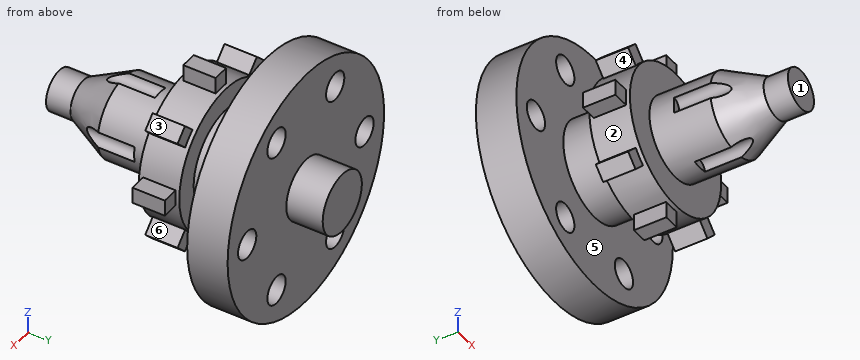
from build123d import *

# Parameters (mm, degrees)
HOLE2_START        = 255
HOLE2_OUTLINE_R    = 17.5
HOLE2_DEPTH        = 50
CIRPATTERN1_COUNT  = 6
RIB2_START         = -20
RIB2_DEPTH         = 40
CIRPATTERN2_COUNT  = 8
SKETCH13_R         = 10
CUT_EXTRUDE1_DEPTH = 125
CIRPATTERN3_COUNT  = 4


# Read off the part's stored shape, not the designer's step: Hole2, Rib2
with BuildPart() as part:
    # Sketch1 → Revolve1 (revolve)
    with BuildSketch(Plane.XY):
        Polygon((0, 0), (0, 350), (37.5, 350), (37.5, 305), (150, 305), (150, 255), (60, 255), (60, 205), (87.5, 205), (87.5, 155), (50, 155), (50, 80), (25, 30), (25, 0), align=None)
    revolve(axis=Axis((0, 0, 0), (0, 1, 0)))

    # Hole2 outline → Hole2 (cut)
    with BuildSketch(Plane(origin=(0, 0, 0), x_dir=(1, 0, 0), z_dir=(0, 1, 0)).offset(HOLE2_START)):
        with Locations((112.5, 0)):
            Circle(HOLE2_OUTLINE_R)
    hole2 = extrude(amount=HOLE2_DEPTH, mode=Mode.SUBTRACT)

    # CirPattern1: Hole2 ×6 about axis
    cirpattern1_axis = Axis((0, 0, 0), (0, 1, 0))
    for i in range(1, CIRPATTERN1_COUNT):
        add(hole2.rotate(cirpattern1_axis, i * 360 / CIRPATTERN1_COUNT), mode=Mode.SUBTRACT)

    # Rib2 outline → Rib2 (add)
    with BuildSketch(Plane(origin=(0, 180, 0), x_dir=(-1, 0, 0), z_dir=(0, -1, 0)).offset(RIB2_START)):
        with BuildLine():
            ThreePointArc((-10, 86.926693254), (0, 87.5), (10, 86.926693254))
            Line((10, 86.926693254), (10, 107.5))
            Line((10, 107.5), (-10, 107.5))
            Line((-10, 107.5), (-10, 86.926693254))
        make_face()
    rib2 = extrude(amount=RIB2_DEPTH)

    # CirPattern2: Rib2 ×8 about axis
    cirpattern2_axis = Axis((0, 0, 0), (0, 1, 0))
    for i in range(1, CIRPATTERN2_COUNT):
        add(rib2.rotate(cirpattern2_axis, i * 360 / CIRPATTERN2_COUNT))

    # Sketch13 → Cut-Extrude1 (cut)
    with BuildSketch(Plane.XZ):
        with Locations((0, 50)):
            Circle(SKETCH13_R)
    cut_extrude1 = extrude(amount=-CUT_EXTRUDE1_DEPTH, mode=Mode.SUBTRACT)

    # CirPattern3: Cut-Extrude1 ×4 about axis
    cirpattern3_axis = Axis((0, 0, 0), (0, 1, 0))
    for i in range(1, CIRPATTERN3_COUNT):
        add(cut_extrude1.rotate(cirpattern3_axis, i * 360 / CIRPATTERN3_COUNT), mode=Mode.SUBTRACT)


solid = part.part
The listing builds one solid part. Answer for the finished solid, in the listing's coordinates (mm). Face numbers are marked on the shaded views. A direction names the side the tool comes from. Give positions to 0.01 mm unless a question says otherwise; leave off trailing zeros. Write each loop counter-clockwise with the first axis right and the second up, starting at its lowest first coordinate (ties: lowest second). Pieces come first, ordered by that corner, then holes. Notation, with made-up numbers: (64, -4) -> (108, -4) arc R22 ccw to (108, 12) -> close; hole circle Ø9 at (-20, 13). An arc over 180 degrees is marked (long way). Use a Markdown table: item, result.
(1) Section C-C, the plane z = 0 is taken. Give the number of separate pieces and of enclosed holes in the cut face, then the cut area to 3 significant figures.
Return value:
| item | result |
|---|---|
| separate pieces | 3 |
| enclosed holes | 0 |
| area | 42,900 mm2 |
(2) Determine the mould class of the marked faces 1, 2 and 3 for opening direction X: released by +X, released by -X, zero draft, split by the parting line, or undercut.
Return value:
| item | result |
|---|---|
| face 1 | zero draft |
| face 2 | undercut |
| face 3 | released by +X |
(3) Flat-ended cylindrical pins translate along their axes: P1, Ø6, axis at x = -94, z = 1, coming from the -Y side; P2, Ø16, axis at x = 3.5, z = -95, coming from the +Y side; P3, Ø6, axis at y = 181, z = -2, coming from the +X side. Find the tip coordinate at first contact, or state that the pin passes through.
Return value:
| item | result |
|---|---|
| P1 | y = 160 |
| P2 | y = 305 |
| P3 | x = 107.5 |
(4) Section A-A, the plane x = -112.5 is taken. Determine the outline of the cut face in (y, z).
Return value:
| item | result |
|---|---|
| outline | (255, -99.22) -> (305, -99.22) -> (305, -17.5) -> (255, -17.5) -> close; (255, 17.5) -> (305, 17.5) -> (305, 99.22) -> (255, 99.22) -> close |
(5) For the marked faces 4, 5 and 6, determine the directions among +Z, -Z, +X, -X, +Y, -Y from which every point of the face is accessible in a straight line to the end or side of a thin tool.
Return value:
| item | result |
|---|---|
| face 4 | -X, -Y |
| face 5 | none |
| face 6 | +X, -Y |
(6) Find the intervals of material crossed by probe 1 along Z at (x, y) = (56, 272); probe 2 along Z at (x, y) = (-57.5, 281.5); probe 3 along Z at (x, y) = (-3.5, 276.5), in increasing order. Write a range as from..to.
Return value:
| item | result |
|---|---|
| probe 1 | -139.15..-114.93, -79.93..79.93, 114.93..139.15 |
| probe 2 | -138.54..-114.88, -79.97..79.97, 114.88..138.54 |
| probe 3 | -149.96..149.96 |
(7) Section D-D, the plane z = -94.5 is taken. Determine the outline of the cut face in (x, y).
Return value:
| item | result |
|---|---|
| outline | (-116.49, 255) -> (-73.5, 255) -> (-73.5, 305) -> (-116.49, 305) -> close; (-39, 255) -> (39, 255) -> (39, 305) -> (-39, 305) -> close; (-10, 160) -> (10, 160) -> (10, 200) -> (-10, 200) -> close; (73.5, 255) -> (116.49, 255) -> (116.49, 305) -> (73.5, 305) -> close |
